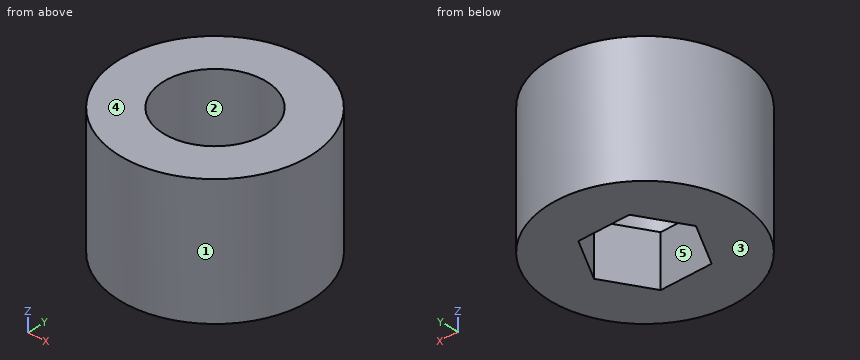
```python
from build123d import *

# Parameters (mm, degrees)
SKETCH_1_R          = 3.7
EXTRUDE_1_DEPTH     = 5
SKETCH_2_R          = 2
CUT_EXTRUDE_1_DEPTH = 3
CUT_EXTRUDE_2_DEPTH = 4


with BuildPart() as part:
    # 草图1 → 凸台-拉伸1 (new body)
    with BuildSketch(Plane.XY):
        Circle(SKETCH_1_R)
    extrude(amount=EXTRUDE_1_DEPTH)

    # 草图2 → 切除-拉伸1 (cut)
    with BuildSketch(Plane.XY.offset(5)):
        Circle(SKETCH_2_R)
    extrude(amount=-CUT_EXTRUDE_1_DEPTH, mode=Mode.SUBTRACT)

    # 草图3 → 切除-拉伸2 (cut)
    with BuildSketch(Plane.XY.offset(2)):
        Polygon((1, -1.732050808), (2, 0), (1, 1.732050808), (-1, 1.732050808), (-2, 0), (-1, -1.732050808), align=None)
    extrude(amount=-CUT_EXTRUDE_2_DEPTH, mode=Mode.SUBTRACT)


solid = part.part
```
Build history of the part. All positions in model axes, mm. Face numbers are marked on the shaded views. A direction names the side the tool comes from. Round coordinates to 2 decimals unless told otherwise and drop trailing zeros. Write each loop counter-clockwise with the first axis right and the second up, starting at its lowest first coordinate (ties: lowest second). Pieces come first, ordered by that corner, then holes.
1) 3-axis set-ups, long thin cutter, end or side, ignore diameter. For the marked faces 4 and 5: which of +Z, -Z, +X, -X, +Y, -Y reach the whole face in a straight line?
2) Drill centre lines: probe 1 along Y at (x, z) = (0, 3.7); probe 2 along Y at (x, z) = (1, 3.7). Where is each one in solid material? Low to high.
3) Band-saw the part on B-B, the plane x = 0. List the corners of the cut face in (y, z), and give its area (3 significant figures).
4) Band-saw the part on C-C, the plane y = -1.5. List the corners of the cut face in (x, z), and give its area (3 significant figures).
5) Mould opens along Y. For the marked faces 1, 2 and 3 say: +Y half, -Y half, draft (parallel to the pull), parting line (faces both ways), or undercut.
6) Pin check, flat tips, straight feed: pin 1 (3 mm diameter, centred on x = -2, z = 2, fed in from +Y); pin 2 (0.5 mm diameter, centred on x = 1.5, y = -1, fed in from +Z); pin 3 (1 mm diameter, centred on y = 2, z = 1.5, fed in from -X). Stop position of each tip, or through.
7) Band-saw the part on A-A, the plane z = 0.7. List the corners of the cut face in (x, y), and give its area (3 significant figures).
8) Band-saw the part on D-D, the plane z = 3.05. List the corners of the cut face in (x, y), and give its area (3 significant figures).
Ans:
1. face 4: +Z, +X, -X, +Y, -Y
1. face 5: +Z, -Z
2. probe 1: y = -3.7 to -2, 2 to 3.7
2. probe 2: y = -3.56 to -1.73, 1.73 to 3.56
3. outline: (-3.7, 0) - (-1.73, 0) - (-1.73, 2) - (-2, 2) - (-2, 5) - (-3.7, 5) - close; (1.73, 0) - (3.7, 0) - (3.7, 5) - (2, 5) - (2, 2) - (1.73, 2) - close
3. area: 18.1 mm2
4. outline: (-3.38, 0) - (-1.13, 0) - (-1.13, 2) - (-1.32, 2) - (-1.32, 5) - (-3.38, 5) - close; (1.13, 0) - (3.38, 0) - (3.38, 5) - (1.32, 5) - (1.32, 2) - (1.13, 2) - close
4. area: 21.3 mm2
5. face 1: parting line
5. face 2: undercut
5. face 3: draft
6. pin 1: stops at y = 3.67
6. pin 2: stops at z = 5
6. pin 3: stops at x = -3.38
7. outline: circle Ø7.4 at (0, 0); hole (-2, 0) - (-1, -1.73) - (1, -1.73) - (2, 0) - (1, 1.73) - (-1, 1.73) - close
7. area: 32.6 mm2
8. outline: circle Ø7.4 at (0, 0); hole circle Ø4 at (0, 0)
8. area: 30.4 mm2
